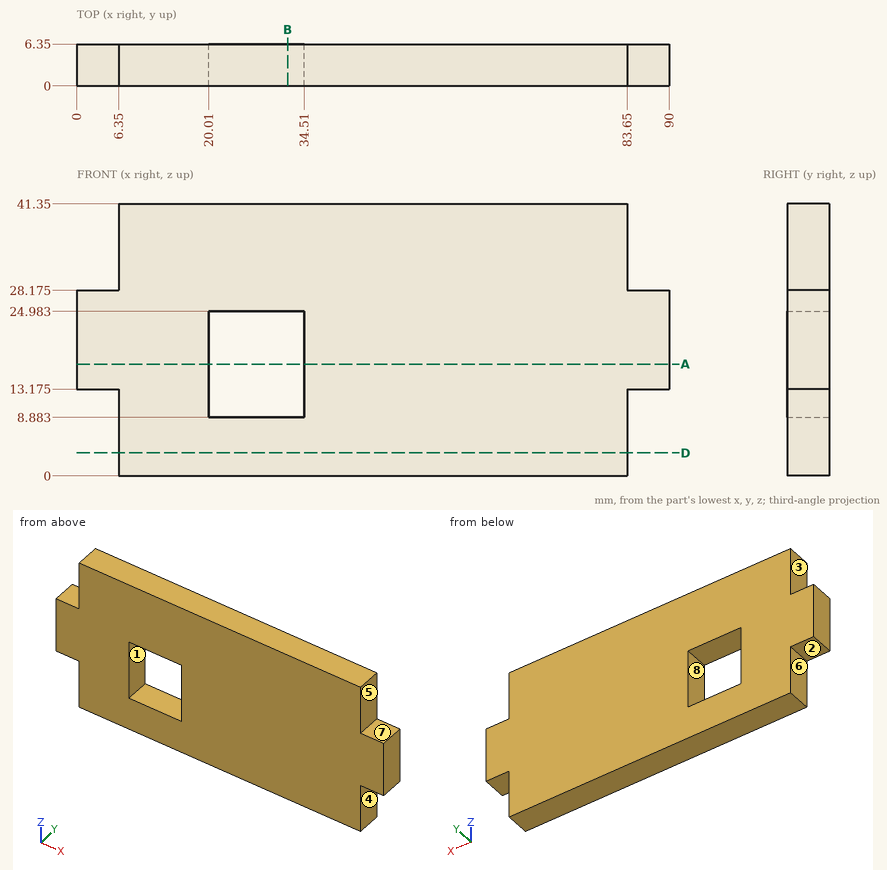
For this review, use the dimensioned drawing (mm, ordinates from the lowest corner) and the shaded views. A direction names the side the tool comes from. Give positions to 0.01 mm unless a question says otherwise; leave off trailing zeros. Write each loop counter-clockwise with the first axis right and the second up, starting at its lowest first coordinate (ties: lowest second). Pieces come first, ordered by that corner, then holes. Notation, with made-up numbers: M 5,8.25 L 62,8.25 A16 cw 62,39.25 Z; hole C 68.5,14 d6. An arc over 180 degrees is marked long. Write item = value, one per line. Start each with the question number.
Q1. We need section D-D (z = 3.5). State the section outline as (x, y) points, plus the area to 3 significant figures.
Q2. We need section B-B (x = 32). State the section outline as (y, z) points, plus the area to 3 significant figures.
Q3. Mouldability with a two-part tool opening along Z and no side actions: class the marked faces 6, 7 and 8 as released by +Z, released by -Z, zero draft, split by the parting line, or undercut.
Q4. For line 1 (Z direction, x = 28, y = 5); line 2 (X direction, y = 2.25, z = 16); line 3 (X direction, y = 2.5, z = 10), list the stretches that pass through material, from the lowest coordinate up.
Q5. Machinability: for the marked faces 1, 2, 3, 4 and 5, which of the approach directions +Z, -Z, +X, -X, +Y, -Y give a long, thin tool a straight path to every point of the face, cutting with its end or side? Answer none if there is none.
Q6. We need section A-A (z = 17). State the section outline as (x, y) points.
Q7. Clearance check with flat-ended pins moving along their axes: pin 1 (1.9 mm diameter, centred on x = 86.5, y = 1.5, fed in from -Z) (3 decimals); pin 2 (3 mm diameter, centred on y = 4, z = 7.5, fed in from -X); pin 3 (3 mm diameter, centred on y = 4.5, z = 34, fed in from +X). State where each tip first meets the part, or that it passes through.
Result set:
q1.outline = M 6.35,0 L 83.65,0 L 83.65,6.35 L 6.35,6.35 Z
q1.area = 491 mm2
q2.outline = M 0,0 L 6.35,0 L 6.35,8.88 L 0,8.88 Z; M 0,24.98 L 6.35,24.98 L 6.35,41.35 L 0,41.35 Z
q2.area = 160 mm2
q3.face_6 = zero draft
q3.face_7 = released by +Z
q3.face_8 = undercut
q4.line_1 = 0 to 8.88, 24.98 to 41.35
q4.line_2 = 0 to 20.01, 34.51 to 90
q4.line_3 = 6.35 to 20.01, 34.51 to 83.65
q5.face_1 = +Y, -Y
q5.face_2 = -Z, -X, +Y, -Y
q5.face_3 = +Z, -X, +Y, -Y
q5.face_4 = -Z, +X, +Y, -Y
q5.face_5 = +Z, +X, +Y, -Y
q6.outline = M 0,0 L 20.01,0 L 20.01,6.35 L 0,6.35 Z; M 34.51,0 L 90,0 L 90,6.35 L 34.51,6.35 Z
q7.pin_1 = 13.175
q7.pin_2 = 6.35
q7.pin_3 = 83.65
